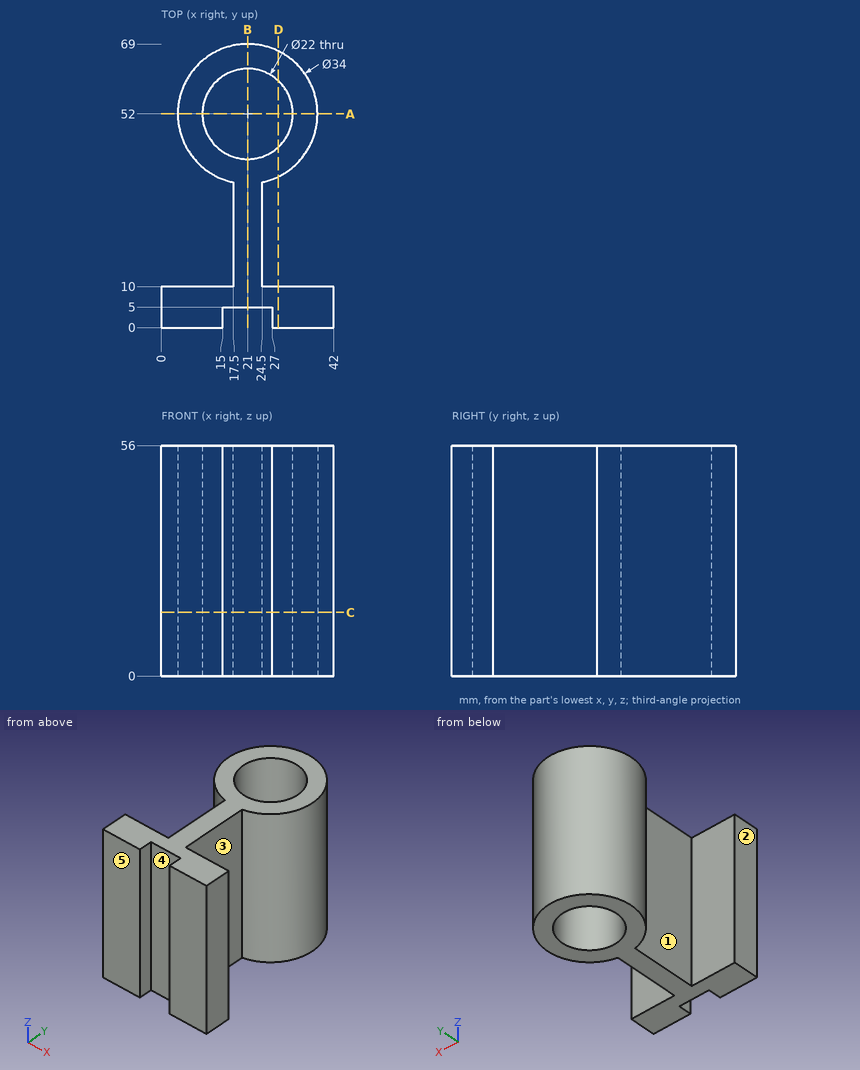
The drawing under review shows one solid part. Ordinate dimensions are in mm from its lowest x, y, z. A direction names the side the tool comes from. Round coordinates to 2 decimals unless told otherwise and drop trailing zeros. Write each loop counter-clockwise with the first axis right and the second up, starting at its lowest first coordinate (ties: lowest second). Pieces come first, ordered by that corner, then holes. Notation, with made-up numbers: (-9.75, 46) - (3.25, 46) arc R18 ccw to (3.25, 74) - close; hole circle Ø7 at (38, -37). An arc over 180 degrees is marked (long way). One line per question, with ' | ' between items.
Item 1: Add section B-B, the plane x = 21. Give the boundary of the cut face in (y, z), then the cut area to 3 significant figures.
Resolved:
outline: (5, 0) - (41, 0) - (41, 56) - (5, 56) - close; (63, 0) - (69, 0) - (69, 56) - (63, 56) - close | area: 2,350 mm2
Item 2: Add section D-D, the plane x = 28.5. Give the boundary of the cut face in (y, z), then the cut area to 3 significant figures.
Resolved:
outline: (0, 0) - (10, 0) - (10, 56) - (0, 56) - close; (36.74, 0) - (43.95, 0) - (43.95, 56) - (36.74, 56) - close; (60.05, 0) - (67.26, 0) - (67.26, 56) - (60.05, 56) - close | area: 1,370 mm2
Item 3: To check wall thickness, follow probe 1 along Y at (x, z) = (21, 35); probe 2 along Y at (x, z) = (14.5, 17); probe 3 along Y at (x, z) = (38.5, 31.5). State the ranges of each line that lie inside material, in increasing order.
Resolved:
probe 1: y = 5 to 41, 63 to 69 | probe 2: y = 0 to 10, 36.29 to 43.13, 60.87 to 67.71 | probe 3: y = 0 to 10
Item 4: Add section A-A, the plane y = 52. Give the boundary of the cut face in (x, z).
Resolved:
outline: (4, 0) - (10, 0) - (10, 56) - (4, 56) - close; (32, 0) - (38, 0) - (38, 56) - (32, 56) - close
Item 5: Add section C-C, the plane z = 15.5. Give the boundary of the cut face in (x, y).
Resolved:
outline: (0, 0) - (15, 0) - (15, 5) - (27, 5) - (27, 0) - (42, 0) - (42, 10) - (24.5, 10) - (24.5, 35.36) arc R17 ccw (long way) to (17.5, 35.36) - (17.5, 10) - (0, 10) - close; hole circle Ø22 at (21, 52)
Item 6: For P1, Ø5, axis at y = 23, z = 39, coming from the +X side; P2, Ø1, axis at y = 20, z = 9.5, coming from the -X side; P3, Ø1, axis at y = 58.5, z = 13, coming from the +X side, all flat-tipped, find the tip position at first contact; note any pin that passes through.
Resolved:
P1: stops at x = 24.5 | P2: stops at x = 17.5 | P3: stops at x = 36.91
Item 7: For the marked faces 1, 2, 3, 4 and 5, list the 3-axis set-ups (+Z, -Z, +X, -X, +Y, -Y) from which the entire face can be reached by the end or side of a thin tool; tool diameter is ignored.
Resolved:
face 1: +Z, -Z, -X | face 2: +Z, -Z, -X, +Y, -Y | face 3: +Z, -Z, +X | face 4: +Z, -Z, -Y | face 5: +Z, -Z, +X, -X, -Y
